from build123d import *

# Parameters (mm, degrees)
SKETCH_W        = 34
SKETCH_H        = 34
PAD_DEPTH       = 80
POCKET_DEPTH    = 80
SKETCH002_R     = 3
POCKET001_DEPTH = 4
SKETCH003_R     = 3
POCKET002_DEPTH = 4
SKETCH004_R     = 4
POCKET003_DEPTH = 2
SKETCH005_R     = 4
POCKET004_DEPTH = 2


with BuildPart() as part:
    # Sketch → Pad (new body)
    with BuildSketch(Plane.XY):
        with Locations((17, 17)):
            Rectangle(SKETCH_W, SKETCH_H)
    extrude(amount=PAD_DEPTH)

    # Sketch001 (on Face6 of Pad) → Pocket (cut)
    with BuildSketch(Plane.XY.offset(80)):
        Polygon((6.5, 27.5), (14, 27.5), (14, 23.5), (17, 21), (20, 23.5), (20, 27.5), (27.5, 27.5), (27.5, 19.5), (23.5, 19.5), (21, 17), (23.5, 14), (27.5, 14), (27.5, 6.5), (20, 6.5), (20, 10.5), (17, 13), (14, 10.5), (14, 6.5), (6.5, 6.5), (6.5, 14), (10.5, 14), (13, 17), (10.5, 19.5), (6.5, 19.5), align=None)
    extrude(amount=-POCKET_DEPTH, mode=Mode.SUBTRACT)

    # Sketch002 (on Face2 of Pocket) → Pocket001 (cut)
    with BuildSketch(Plane(origin=(0, 0, 0), x_dir=(0, -1, 0), z_dir=(-1, 0, 0))):
        with Locations((-17, 60)):
            Circle(SKETCH002_R)
        with Locations((-17, 20)):
            Circle(SKETCH002_R)
    extrude(amount=-POCKET001_DEPTH, mode=Mode.SUBTRACT)

    # Sketch003 (on Face3 of Pocket001) → Pocket002 (cut)
    with BuildSketch(Plane.YZ.offset(34)):
        with Locations((17, 60)):
            Circle(SKETCH003_R)
        with Locations((17, 20)):
            Circle(SKETCH003_R)
    extrude(amount=-POCKET002_DEPTH, mode=Mode.SUBTRACT)

    # Sketch004 (on Face1 of Pocket002) → Pocket003 (cut)
    with BuildSketch(Plane(origin=(0, 34, 0), x_dir=(-1, 0, 0), z_dir=(0, 1, 0))):
        with Locations((-27, 60)):
            Circle(SKETCH004_R)
        with Locations((-7, 60)):
            Circle(SKETCH004_R)
        with Locations((-27, 20)):
            Circle(SKETCH004_R)
        with Locations((-7, 20)):
            Circle(SKETCH004_R)
    extrude(amount=-POCKET003_DEPTH, mode=Mode.SUBTRACT)

    # Sketch005 (on Face10 of Pocket003) → Pocket004 (cut)
    with BuildSketch(Plane.XZ):
        with Locations((7, 60)):
            Circle(SKETCH005_R)
        with Locations((27, 60)):
            Circle(SKETCH005_R)
        with Locations((7, 20)):
            Circle(SKETCH005_R)
        with Locations((27, 20)):
            Circle(SKETCH005_R)
    extrude(amount=-POCKET004_DEPTH, mode=Mode.SUBTRACT)


solid = part.part
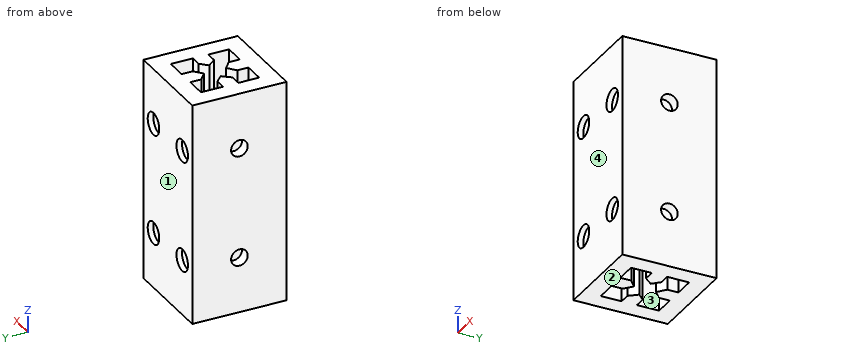
Verification items for the finished model (mm, model axes). Face numbers are marked on the shaded views. Coordinates: 2 decimals unless noted, no trailing zeros. Order: outer loops, then holes, each group sorted by start corner. A loop starts at its lowest first (then second) coordinate and runs counter-clockwise, first axis right, second up. Notation, with made-up numbers: M 27,43.25 L 47,43.25 A9 cw 47,57.25 Z; hole C 50.5,39 d4. An arc over 180 degrees is marked long. One line per item, written item: value. Start each with the question number.
Item 1: Mould release check, pull along Y, two halves, no side actions. Record for the marked faces 1, 2, 3 and 4: released by +Y, released by -Y, zero draft, split by the parting line, or undercut.
Item 2: Scan lines: probe 1 along Z at (x, y) = (2.6, 17); probe 2 along Z at (x, y) = (7, 33); probe 3 along X at (y, z) = (24.5, 57). Record each from-to range of solid material in increasing order.
Item 3: Sectioned sample at A-A (x = 22). Enter the section's corners in (y, z), then the cut area to 3 significant figures.
Item 4: Sectioned sample at C-C (z = 69.5). Enter the section's corners in (x, y).
Item 5: Sectioned sample at B-B (y = 15). Enter the section's corners in (x, z), then the cut area to 3 significant figures.
Item 6: Sectioned sample at D-D (x = 9). Enter the section's corners in (y, z).
Item 7: Gauge pin test, flat ends, axial feed: pin 1 (7 mm diameter, centred on x = 7, z = 20, fed in from -Y); pin 2 (6.5 mm diameter, centred on x = 7, z = 60, fed in from +Y); pin 3 (1.8 mm diameter, centred on y = 18, z = 58.5, fed in from +X). Record the tip position at first contact, or that the pin passes through.
Conclusion:
1. face 1: released by +Y
1. face 2: zero draft
1. face 3: undercut
1. face 4: released by -Y
2. probe 1: z = 0 to 17, 23 to 57, 63 to 80
2. probe 2: z = 0 to 16, 24 to 56, 64 to 80
2. probe 3: x = 0 to 6.5, 14 to 20, 27.5 to 34
3. outline: M 0,0 L 6.5,0 L 6.5,80 L 0,80 Z; M 15.8,0 L 18,0 L 18,80 L 15.8,80 Z; M 27.5,0 L 34,0 L 34,80 L 27.5,80 Z
3. area: 1,220 mm^2
4. outline: M 0,0 L 34,0 L 34,34 L 0,34 Z; hole M 6.5,6.5 L 14,6.5 L 14,10.5 L 17,13 L 20,10.5 L 20,6.5 L 27.5,6.5 L 27.5,14 L 23.5,14 L 21,17 L 23.5,19.5 L 27.5,19.5 L 27.5,27.5 L 20,27.5 L 20,23.5 L 17,21 L 14,23.5 L 14,27.5 L 6.5,27.5 L 6.5,19.5 L 10.5,19.5 L 13,17 L 10.5,14 L 6.5,14 Z
5. outline: M 0,0 L 11.33,0 L 11.33,80 L 0,80 L 0,62.24 L 4,62.24 L 4,57.76 L 0,57.76 L 0,22.24 L 4,22.24 L 4,17.76 L 0,17.76 Z; M 22.67,0 L 34,0 L 34,17.76 L 30,17.76 L 30,22.24 L 34,22.24 L 34,57.76 L 30,57.76 L 30,62.24 L 34,62.24 L 34,80 L 22.67,80 Z
5. area: 1,740 mm^2
6. outline: M 0,0 L 6.5,0 L 6.5,80 L 0,80 L 0,63.46 L 2,63.46 L 2,56.54 L 0,56.54 L 0,23.46 L 2,23.46 L 2,16.54 L 0,16.54 Z; M 14,0 L 19.5,0 L 19.5,80 L 14,80 Z; M 27.5,0 L 34,0 L 34,16.54 L 32,16.54 L 32,23.46 L 34,23.46 L 34,56.54 L 32,56.54 L 32,63.46 L 34,63.46 L 34,80 L 27.5,80 Z
7. pin 1: stops at y = 2
7. pin 2: stops at y = 32
7. pin 3: stops at x = 30
